```python
from build123d import *

# Parameters (mm, degrees)
BOSS_EXTRU_1_DEPTH      = 2
ESQUISSE2_R             = 2.25
ENL_V_MAT_EXTRU_1_DEPTH = 3
ENL_V_MAT_EXTRU_2_DEPTH = 10


with BuildPart() as part:
    # Esquisse1 → Boss.-Extru.1 (new body)
    with BuildSketch(Plane.XY):
        with BuildLine():
            Line((35, -45), (-35, -45))
            ThreePointArc((-35, -45), (-42.071067812, -42.071067812), (-45, -35))
            Line((-45, -35), (-45, 35))
            ThreePointArc((-45, 35), (-42.071067812, 42.071067812), (-35, 45))
            Line((-35, 45), (35, 45))
            ThreePointArc((35, 45), (42.071067812, 42.071067812), (45, 35))
            Line((45, 35), (45, -35))
            ThreePointArc((45, -35), (42.071067812, -42.071067812), (35, -45))
        make_face()
    extrude(amount=BOSS_EXTRU_1_DEPTH)

    # Esquisse2 → Enlèv. mat.-Extru.1 (cut, through all)
    with BuildSketch(Plane(origin=(0, 0, 0), x_dir=(-1, 0, 0), z_dir=(0, 0, -1))):
        with Locations((-35, -35)):
            Circle(ESQUISSE2_R)
        with Locations((-35, 35)):
            Circle(ESQUISSE2_R)
        with Locations((35, -35)):
            Circle(ESQUISSE2_R)
        with Locations((35, 35)):
            Circle(ESQUISSE2_R)
    extrude(amount=-ENL_V_MAT_EXTRU_1_DEPTH, mode=Mode.SUBTRACT)

    # Esquisse4 → Enlèv. mat.-Extru.2 (cut)
    with BuildSketch(Plane(origin=(0, 0, 0), x_dir=(-1, 0, 0), z_dir=(0, 0, -1))):
        with BuildLine():
            Line((-18.471463814, -28.745227889), (18.471463814, -28.745227889))
            ThreePointArc((18.471463814, -28.745227889), (25.542531626, -25.816295701), (28.471463814, -18.745227889))
            Line((28.471463814, -18.745227889), (28.471463814, 18.745227889))
            ThreePointArc((28.471463814, 18.745227889), (25.542531626, 25.816295701), (18.471463814, 28.745227889))
            Line((18.471463814, 28.745227889), (-18.471463814, 28.745227889))
            ThreePointArc((-18.471463814, 28.745227889), (-25.542531626, 25.816295701), (-28.471463814, 18.745227889))
            Line((-28.471463814, 18.745227889), (-28.471463814, -18.745227889))
            ThreePointArc((-28.471463814, -18.745227889), (-25.542531626, -25.816295701), (-18.471463814, -28.745227889))
        make_face()
    extrude(amount=-ENL_V_MAT_EXTRU_2_DEPTH, mode=Mode.SUBTRACT)


solid = part.part
```
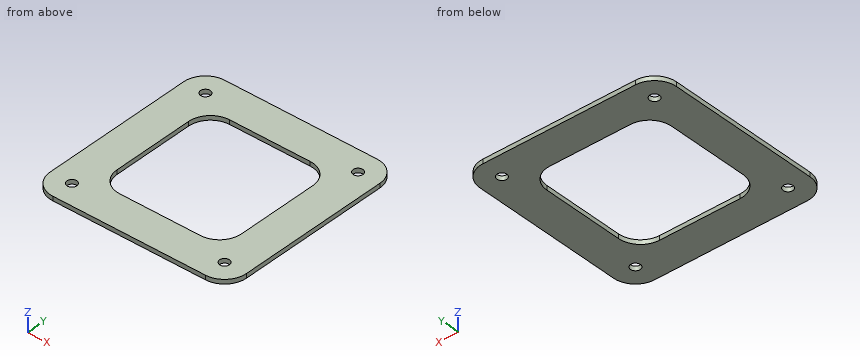
Can you work these out from the model? Positions are in its coordinate system, mm. Round coordinates to 2 decimals unless told otherwise and drop trailing zeros. Loops run counter-clockwise (first coordinate to the right, second up) from the corner with the lowest first, then second, coordinate; pieces in that order, holes last. Notation, with made-up numbers: (58, 65.5) -> (105, 65.5) arc R20 ccw to (105, 79.5) -> close; hole circle Ø6 at (59, -6). An arc over 180 degrees is marked (long way). Answer in a Markdown table with one row per item.
Item 1: If I drill on probe 1 along Y at (x, z) = (35, 1.2); probe 2 along X at (y, z) = (-3, 1.5); probe 3 along Y at (x, z) = (18, 1.7), over which ranges is the centre line in solid material (lowest first)?
Answer block:
| item | result |
|---|---|
| probe 1 | -45 to -37.25, -32.75 to 32.75, 37.25 to 45 |
| probe 2 | -45 to -28.47, 28.47 to 45 |
| probe 3 | -45 to -28.75, 28.75 to 45 |
Item 2: Suppose I cut it at A-A, the plane x = -2. List the corners of the cut face in (y, z) for me, plus the area to 3 significant figures.
Answer block:
| item | result |
|---|---|
| outline | (-45, 0) -> (-28.75, 0) -> (-28.75, 2) -> (-45, 2) -> close; (28.75, 0) -> (45, 0) -> (45, 2) -> (28.75, 2) -> close |
| area | 65.0 mm² |
Item 3: Suppose I cut it at B-B, the plane y = 17. List the corners of the cut face in (x, z) for me, plus the area to 3 significant figures.
Answer block:
| item | result |
|---|---|
| outline | (-45, 0) -> (-28.47, 0) -> (-28.47, 2) -> (-45, 2) -> close; (28.47, 0) -> (45, 0) -> (45, 2) -> (28.47, 2) -> close |
| area | 66.1 mm² |
Item 4: Suppose I cut it at C-C, the plane z = 0.9. List the corners of the cut face in (x, y) for me, plus the area to 3 significant figures.
Answer block:
| item | result |
|---|---|
| outline | (-45, -35) arc R10 ccw to (-35, -45) -> (35, -45) arc R10 ccw to (45, -35) -> (45, 35) arc R10 ccw to (35, 45) -> (-35, 45) arc R10 ccw to (-45, 35) -> close; hole circle Ø4.5 at (-35, -35); hole circle Ø4.5 at (-35, 35); hole (-28.47, -18.75) arc R10 ccw to (-18.47, -28.75) -> (18.47, -28.75) arc R10 ccw to (28.47, -18.75) -> (28.47, 18.75) arc R10 ccw to (18.47, 28.75) -> (-18.47, 28.75) arc R10 ccw to (-28.47, 18.75) -> close; hole circle Ø4.5 at (35, -35); hole circle Ø4.5 at (35, 35) |
| area | 4,760 mm² |
